Here's how the part is built. I have some questions about the finished solid (model axes, mm). A direction names the side the tool comes from. Give positions to 0.01 mm unless a question says otherwise; leave off trailing zeros. Write each loop counter-clockwise with the first axis right and the second up, starting at its lowest first coordinate (ties: lowest second). Pieces come first, ordered by that corner, then holes. Notation, with made-up numbers: (38, -32) - (92, -32) arc R26 cw to (92, -18) - close; hole circle Ø8 at (75.5, -3.75). An arc over 180 degrees is marked (long way). Use a Markdown table: item, result.
```python
from build123d import *

# Parameters (mm, degrees)
F0_W     = 81.6473141313
F0_H     = 80.3374648094
F1_DEPTH = 38.1
F3_DEPTH = 76.2


# Not quite as in the source:
# - the program builds the solid bodies; features that only make, move or delete a surface that nothing else refers to are left out


with BuildPart() as f1:
    # F0 (on Top) → F1 (new body)
    with BuildSketch(Plane.XY):
        Rectangle(F0_W, F0_H)
        Polygon((-15.8581690014, 11.5216341958), (-6.0572815592, 18.6423957348), (6.0572815592, 18.6423957348), (15.8581690014, 11.5216341958), (19.6017748844, 0), (15.8581690014, -11.5216341958), (6.0572815592, -18.6423957348), (-6.0572815592, -18.6423957348), (-15.8581690014, -11.5216341958), (-19.6017748844, 0), align=None, mode=Mode.SUBTRACT)
    extrude(amount=F1_DEPTH)

    # F0 (on Top) → F3 (join)
    with BuildSketch(Plane.XY):
        Polygon((6.0572815592, 18.6423957348), (-6.0572815592, 18.6423957348), (-15.8581690014, 11.5216341958), (-19.6017748844, 0), (-15.8581690014, -11.5216341958), (-6.0572815592, -18.6423957348), (6.0572815592, -18.6423957348), (15.8581690014, -11.5216341958), (19.6017748844, 0), (15.8581690014, 11.5216341958), align=None)
    extrude(amount=F3_DEPTH)


solid = f1.part
```
Item 1: If we section it at B-B, the plane x = -0.5: Write out the boundary of the cut face in (y, z), plus the area to 3 significant figures.
Values:
| item | result |
|---|---|
| outline | (-40.17, 0) - (40.17, 0) - (40.17, 38.1) - (18.64, 38.1) - (18.64, 76.2) - (-18.64, 76.2) - (-18.64, 38.1) - (-40.17, 38.1) - close |
| area | 4,480 mm2 |
Item 2: For faces 1 (the flat face through (-10.89, 15.13, 56.88)), 2 (the flat face through (10.89, -15.13, 56.88)), 3 (the flat face through (11.03, 15.03, 56.88)), which set-ups out of +Z, -Z, +X, -X, +Y, -Y let a thin tool reach every point of the face, with its end or its side?
Values:
| item | result |
|---|---|
| face 1 | +Z, -X, +Y |
| face 2 | +Z, +X, -Y |
| face 3 | +Z, +X, +Y |
Item 3: If we section it at A-A, the plane z = 58: Write out the boundary of the cut face in (x, y).
Values:
| item | result |
|---|---|
| outline | (-19.6, 0) - (-15.86, -11.52) - (-6.06, -18.64) - (6.06, -18.64) - (15.86, -11.52) - (19.6, 0) - (15.86, 11.52) - (6.06, 18.64) - (-6.06, 18.64) - (-15.86, 11.52) - close |
Item 4: If we section it at C-C, the plane y = 29.5: Write out the boundary of the cut face in (x, z), plus the area to 3 significant figures.
Values:
| item | result |
|---|---|
| outline | (-40.82, 0) - (40.82, 0) - (40.82, 38.1) - (-40.82, 38.1) - close |
| area | 3,110 mm2 |
Item 5: I need wall thicknesses on line 1 along Z through (x, y) = (23.5, 26); line 2 along Y through (x, z) = (3, 53); line 3 along X through (y, z) = (18.5, 55.5). Which ranges of each line are inside material? Lowest first, please. Write a range as [from, to].
Values:
| item | result |
|---|---|
| line 1 | z = [0, 38.1] |
| line 2 | y = [-18.64, 18.64] |
| line 3 | x = [-6.25, 6.25] |
Item 6: If we section it at D-D, the plane x = 13: Write out the boundary of the cut face in (y, z), plus the area to 3 significant figures.
Values:
| item | result |
|---|---|
| outline | (-40.17, 0) - (40.17, 0) - (40.17, 38.1) - (13.6, 38.1) - (13.6, 76.2) - (-13.6, 76.2) - (-13.6, 38.1) - (-40.17, 38.1) - close |
| area | 4,100 mm2 |
Item 7: Will these pins go through, and if not, where does the flat tip stop? pin 1 Ø1.5 at (x, y) = (28.5, -18) entering from -Z; pin 2 Ø6 at (x, z) = (-2.5, 50.5) entering from +Y; pin 3 Ø3.5 at (x, z) = (0.5, 48.5) entering from -Y; pin 4 Ø1.5 at (y, z) = (-1, 45.5) entering from +X.
Values:
| item | result |
|---|---|
| pin 1 | stops at z = 0 |
| pin 2 | stops at y = 18.64 |
| pin 3 | stops at y = -18.64 |
| pin 4 | stops at x = 19.52 |
